Check sheet for the modelled part. Datum: model origin and axes. Units: mm. A direction names the side the tool comes from. Round coordinates to 2 decimals unless told otherwise and drop trailing zeros. Order: outer loops, then holes, each group sorted by start corner. A loop starts at its lowest first (then second) coordinate and runs counter-clockwise, first axis right, second up.
Q1. Scan lines: probe 1 along Y at (x, z) = (0.25, -7.25); probe 2 along X at (y, z) = (-20, -2.25); probe 3 along Z at (x, y) = (-0.25, -21). Record each from-to range of solid material in increasing order.
Q2. Cross-section at A-A on y = 5. Record the cut outline in (x, z).
Q3. Set-up check for faces 1 (the flat face through (0, 15.916, -2)), 2 (the flat face through (-4.5, 14.764, -3.4)), 3 (the flat face through (-1.4, -33.236, -6)): record each of +Z, -Z, +X, -X, +Y, -Y from which the full face is reachable in a straight line by a thin tool's end or side.
Q4. Depth check by flat-ended pin: P1, Ø5, axis at y = -1.5, z = -6, coming from the -X side; P2, Ø1, axis at x = -1, y = -26, coming from the +Z side; P3, Ø1.5, axis at y = -23.5, z = 0, coming from the +X side. Enter the tip coordinate at first touch or a pass-through.
from build123d import *

# Parameters (mm, degrees)
REDONDEO1_R = 0.5


with BuildPart() as part:
    # Croquis2 → Revolución1 (revolve)
    with BuildSketch(Plane(origin=(0, 0, 0), x_dir=(0, 0, -1), z_dir=(1, 0, 0))):
        Polygon((2.083734943, 15.916127666), (4.583734943, 15.916127666), (4.583734943, 14.916127666), (6.583734943, 14.763533095), (8.583734943, 14.763533095), (8.583734943, -33.236466905), (6.083734943, -33.236466905), (6.083734943, -34.236466905), (2.083734943, -34.236466905), align=None)
    revolve(axis=Axis((0, -34.236466905, -2.083734943), (0, 1, 0)))

    # Redondeo1
    redondeo1_edges = [part.edges().sort_by_distance(p)[0] for p in [
        (0, -34.236466905, 1.916265057),
        (0, -33.236466905, 4.416265057),
        (0, 14.763533095, 4.416265057),
        (0, 14.916127666, 0.416265057),
        (0, 15.916127666, 0.416265057),
    ]]
    fillet(redondeo1_edges, radius=REDONDEO1_R)


solid = part.part
Results found:
1. probe 1: y = -33.24 to 14.76
1. probe 2: x = -6.5 to 6.5
1. probe 3: z = -8.58 to 4.41
2. outline: circle Ø13 at (0, -2.08)
3. face 1: +Z, -Z, +X, -X, +Y
3. face 2: +Y
3. face 3: -Y
4. P1: stops at x = -6.34
4. P2: stops at z = 4.4
4. P3: stops at x = 6.36
